from build123d import *

# Parameters (mm, degrees)
SKETCH1_R           = 2.5
BOSS_EXTRUDE1_DEPTH = 15
SKETCH2_R           = 2.5
CUT_EXTRUDE1_DEPTH  = 20


with BuildPart() as part:
    # Sketch1 → Boss-Extrude1 (new body)
    with BuildSketch(Plane(origin=(0, 0, 0), x_dir=(1, 0, 0), z_dir=(0, 1, 0))):
        with BuildLine():
            Line((-59.967506742, 33.972160861), (59.967506742, 33.972160861))
            ThreePointArc((59.967506742, 33.972160861), (61.305448214, 33.78982758), (62.545809183, 33.256125908))
            Line((62.545809183, 33.256125908), (122.57830244, -2.874403203))
            ThreePointArc((122.57830244, -2.874403203), (124.283965047, -9.736670691), (117.42169756, -11.442333298))
            Line((117.42169756, -11.442333298), (59.768652626, 23.256125908))
            ThreePointArc((59.768652626, 23.256125908), (58.528291658, 23.78982758), (57.190350186, 23.972160861))
            Line((57.190350186, 23.972160861), (-57.190350186, 23.972160861))
            ThreePointArc((-57.190350186, 23.972160861), (-58.528291658, 23.78982758), (-59.768652626, 23.256125908))
            Line((-59.768652626, 23.256125908), (-117.42169756, -11.442333298))
            ThreePointArc((-117.42169756, -11.442333298), (-124.283965047, -9.736670691), (-122.57830244, -2.874403203))
            Line((-122.57830244, -2.874403203), (-62.545809183, 33.256125908))
            ThreePointArc((-62.545809183, 33.256125908), (-61.305448214, 33.78982758), (-59.967506742, 33.972160861))
        make_face()
        with Locations(Location((-120, -7.158368251, 0), (0, 0, 270))):
            Circle(SKETCH1_R, mode=Mode.SUBTRACT)
        with Locations(Location((120, -7.158368251, 0), (0, 0, 90))):
            Circle(SKETCH1_R, mode=Mode.SUBTRACT)
    extrude(amount=BOSS_EXTRUDE1_DEPTH)

    # Sketch2 → Cut-Extrude1 (cut)
    with BuildSketch(Plane(origin=(0, 15, 0), x_dir=(1, 0, 0), z_dir=(0, 1, 0))):
        with Locations(Location((0, 28.972160861, 0), (0, 0, 270))):
            Circle(SKETCH2_R)
    extrude(amount=-CUT_EXTRUDE1_DEPTH, mode=Mode.SUBTRACT)


solid = part.part
CAD build for the part. Positions are in the model's coordinates, mm. A direction names the side the tool comes from. Give positions to 0.01 mm unless a question says otherwise; leave off trailing zeros. Order: outer loops, then holes, each group sorted by start corner. A loop starts at its lowest first (then second) coordinate and runs counter-clockwise, first axis right, second up. Notation, with made-up numbers: (60, 36) -> (101, 36) arc R28 ccw to (101, 72) -> close; hole circle Ø1 at (79.25, 41.5). An arc over 180 degrees is marked (long way). Return JSON: item names as keys, results as strings.
Q1. Mould opens along Z. For faces 1 (the face through (-0.958, 7.605, -26.663)), 2 (the face through (124.34, 7.4, 9.64)), 3 (the face through (88.999, 7.395, -5.664)) say: pulls with the +Z half, pulls with the -Z half, needs draft (parallel to the pull), parting line crosses it, or undercut.
Working result:
{"face 1": "undercut", "face 2": "parting line crosses it", "face 3": "pulls with the +Z half"}
Q2. Saw through at B-B (y = 2.5). Write the cut outline in (x, z).
Working result:
{"outline": "(-122.58, 2.87) -> (-62.55, -33.26) arc R5 ccw to (-59.97, -33.97) -> (59.97, -33.97) arc R5 ccw to (62.55, -33.26) -> (122.58, 2.87) arc R5 ccw to (117.42, 11.44) -> (59.77, -23.26) arc R5 cw to (57.19, -23.97) -> (-57.19, -23.97) arc R5 cw to (-59.77, -23.26) -> (-117.42, 11.44) arc R5 ccw to start; hole circle Ø5 at (-120, 7.16); hole circle Ø5 at (0, -28.97); hole circle Ø5 at (120, 7.16)"}
Q3. Saw through at A-A (x = 0). Write the cut outline in (y, z), then the cut area to 3 significant figures.
Working result:
{"outline": "(0, -33.97) -> (15, -33.97) -> (15, -31.47) -> (0, -31.47) -> close; (0, -26.47) -> (15, -26.47) -> (15, -23.97) -> (0, -23.97) -> close", "area": "75.0 mm²"}
Q4. Flat gauge pins, fed straight in: pin 1 (1 mm diameter, centred on y = 10.5, z = -6, fed in from +X); pin 2 (6 mm diameter, centred on x = -120, z = 7.16, fed in from +Y); pin 3 (2 mm diameter, centred on x = 91, y = 12.5, fed in from -Z); pin 4 (7.5 mm diameter, centred on x = -25.5, y = 6, fed in from +Z). Where does each tip first touch, or does it go through?
Working result:
{"pin 1": "x = 108.66", "pin 2": "y = 15", "pin 3": "z = -16.73", "pin 4": "z = -23.97"}
Q5. Saw through at C-C (z = -5). Write the cut outline in (x, y).
Working result:
{"outline": "(-109.49, 0) -> (-90.1, 0) -> (-90.1, 15) -> (-109.49, 15) -> close; (90.1, 0) -> (109.49, 0) -> (109.49, 15) -> (90.1, 15) -> close"}
Q6. Saw through at D-D (z = 7). Write the cut outline in (x, y), then the cut area to 3 significant figures.
Working result:
{"outline": "(-125, 0) -> (-122.49, 0) -> (-122.49, 15) -> (-125, 15) -> close; (-117.51, 0) -> (-110.04, 0) -> (-110.04, 15) -> (-117.51, 15) -> close; (110.04, 0) -> (117.51, 0) -> (117.51, 15) -> (110.04, 15) -> close; (122.49, 0) -> (125, 0) -> (125, 15) -> (122.49, 15) -> close", "area": "299 mm²"}
Q7. Which spindle directions (+Z, -Z, +X, -X, +Y, -Y) get a long thin tool onto all of the face, cutting with end or side? Do faces 4 (the face through (1, 7, -23.972)), 5 (the face through (92.142, 7.395, -15.444)). Say none if no direction does.
Working result:
{"face 4": "+Z, +Y, -Y", "face 5": "-Z, +X, +Y, -Y"}
Q8. Drill centre lines: line 1 (X direction, y = 2, z = 9); line 2 (X direction, y = 8, z = -14); line 3 (X direction, y = 2, z = -22). Where is each one in solid material? Low to high.
Working result:
{"line 1": "-124.65 to -121.69, -118.31 to -113.36, 113.36 to 118.31, 121.69 to 124.65", "line 2": "-94.54 to -75.15, 75.15 to 94.54", "line 3": "-81.25 to -61.86, 61.86 to 81.25"}
